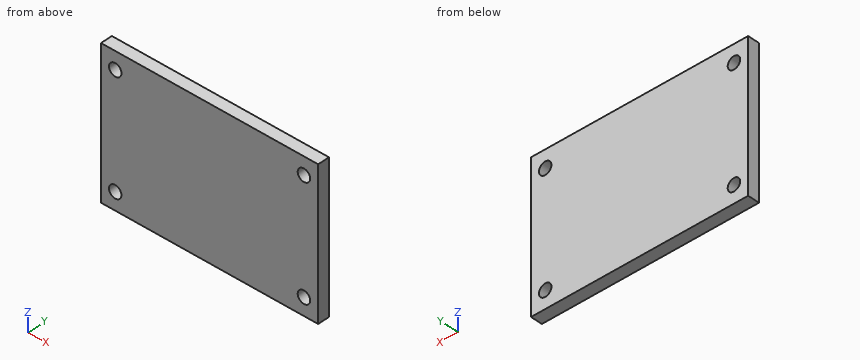
from build123d import *

# Parameters (mm, degrees)
SKETCH1_W                = 55.8
SKETCH1_H                = 37.6
BOSS_EXTRUDE1_DEPTH      = 3
M3_CLEARANCE_HOLE1_D     = 3.2
M3_CLEARANCE_HOLE1_DEPTH = 3


with BuildPart() as part:
    # Sketch1 → Boss-Extrude1 (new body)
    with BuildSketch(Plane(origin=(0, 0, 0), x_dir=(1, 0, 0), z_dir=(0, 1, 0))):
        with Locations((27.9, 18.8)):
            Rectangle(SKETCH1_W, SKETCH1_H)
    extrude(amount=BOSS_EXTRUDE1_DEPTH)

    # M3 Clearance Hole1
    with Locations(Plane(origin=(0, 3, 0), x_dir=(1, 0, 0), z_dir=(0, 1, 0))):
        with Locations((3.65, 33.15), (52.15, 33.15), (52.15, 4.45), (3.65, 4.45)):
            Hole(M3_CLEARANCE_HOLE1_D / 2, depth=M3_CLEARANCE_HOLE1_DEPTH)


solid = part.part
Part model, mm, in its own coordinate system. Give positions to 0.01 mm unless a question says otherwise; leave off trailing zeros. Order: outer loops, then holes, each group sorted by start corner. A loop starts at its lowest first (then second) coordinate and runs counter-clockwise, first axis right, second up. Notation, with made-up numbers: (11.5, -11.5) -> (21.5, -11.5) arc R6 cw to (21.5, -5.5) -> close; hole circle Ø11 at (85, -39.75). An arc over 180 degrees is marked (long way). Use one line per item in the form item = value.
(1) Saw through at A-A (x = 52.15). Write the cut outline in (y, z), then the cut area to 3 significant figures.
Solution:
outline = (0, -37.6) -> (3, -37.6) -> (3, -34.75) -> (0, -34.75) -> close; (0, -31.55) -> (3, -31.55) -> (3, -6.05) -> (0, -6.05) -> close; (0, -2.85) -> (3, -2.85) -> (3, 0) -> (0, 0) -> close
area = 93.6 mm²
(2) Drill centre lines: line 1 (X direction, y = 1.05, z = -4.45); line 2 (Z direction, x = 3.65, y = 1.9); line 3 (X direction, y = 1, z = -32.5). Where is each one in solid material? Low to high. Write a range as from..to.
Solution:
line_1 = 0..2.05, 5.25..50.55, 53.75..55.8
line_2 = -37.6..-34.75, -31.55..-6.05, -2.85..0
line_3 = 0..2.19, 5.11..50.69, 53.61..55.8
(3) Saw through at B-B (z = -33.15). Write the cut outline in (x, y), then the cut area to 3 significant figures.
Solution:
outline = (0, 0) -> (2.05, 0) -> (2.05, 3) -> (0, 3) -> close; (5.25, 0) -> (50.55, 0) -> (50.55, 3) -> (5.25, 3) -> close; (53.75, 0) -> (55.8, 0) -> (55.8, 3) -> (53.75, 3) -> close
area = 148 mm²
(4) Saw through at C-C (y = 1.3). Write the cut outline in (x, z).
Solution:
outline = (0, -37.6) -> (55.8, -37.6) -> (55.8, 0) -> (0, 0) -> close; hole circle Ø3.2 at (3.65, -33.15); hole circle Ø3.2 at (3.65, -4.45); hole circle Ø3.2 at (52.15, -33.15); hole circle Ø3.2 at (52.15, -4.45)
